from build123d import *

# Parameters (mm, degrees)
SKETCH_R           = 0.75
SKETCH_R_2         = 0.6
PAD_DEPTH          = 4.8
PAD_DEPTH_BACK     = 0.8
SKETCH001_R        = 3.5
SKETCH001_R_2      = 0.6
PAD001_DEPTH       = 0.8
POCKET_DEPTH       = 24.348308
POLARPATTERN_COUNT = 4
SKETCH003_R        = 1.5
SKETCH003_R_2      = 0.6
PAD002_DEPTH       = 0.2


with BuildPart() as part:
    # Sketch → Pad (new body, two sides)
    with BuildSketch(Plane.XY) as pad_sk:
        Circle(SKETCH_R)
        Circle(SKETCH_R_2, mode=Mode.SUBTRACT)
    extrude(amount=PAD_DEPTH)
    extrude(pad_sk.sketch, amount=-PAD_DEPTH_BACK)

    # Sketch001 → Pad001 (join)
    with BuildSketch(Plane.XY):
        Circle(SKETCH001_R)
        Circle(SKETCH001_R_2, mode=Mode.SUBTRACT)
    extrude(amount=PAD001_DEPTH)

    # Sketch002 (on Face8 of Pad001) → Pocket (cut, through all)
    with BuildSketch(Plane.XY.offset(0.8)):
        with BuildLine():
            Line((-0.5, 3.75), (0.5, 3.75))
            Line((0.5, 3.75), (0.5, 2.25))
            ThreePointArc((-0.5, 2.25), (0, 1.75), (0.5, 2.25))
            Line((-0.5, 2.25), (-0.5, 3.75))
        make_face()
    pocket = extrude(amount=-POCKET_DEPTH, mode=Mode.SUBTRACT)

    # PolarPattern: Pocket ×4 about axis
    polarpattern_axis = Axis((0, 0, 0.8), (0, 0, 1))
    for i in range(1, POLARPATTERN_COUNT):
        add(pocket.rotate(polarpattern_axis, i * 360 / POLARPATTERN_COUNT), mode=Mode.SUBTRACT)

    # Sketch003 (on Face23 of PolarPattern) → Pad002 (join)
    with BuildSketch(Plane.XY.offset(0.8)):
        Circle(SKETCH003_R)
        Circle(SKETCH003_R_2, mode=Mode.SUBTRACT)
    extrude(amount=PAD002_DEPTH)


solid = part.part
Geometry check sheet. Reference: the model listing, model coordinates, mm. A direction names the side the tool comes from. Round coordinates to 2 decimals unless told otherwise and drop trailing zeros. Loops run counter-clockwise (first coordinate to the right, second up) from the corner with the lowest first, then second, coordinate; pieces in that order, holes last. Notation, with made-up numbers: (58.5, 68) - (109.5, 68) arc R23 ccw to (109.5, 79) - close; hole circle Ø7 at (58.25, -2). An arc over 180 degrees is marked (long way). One line per question, with ' | ' between items. Start each with the question number.
1. Depth check by flat-ended pin: pin 1 (1 mm diameter, centred on x = 1, z = 3, fed in from -Y); pin 2 (0.6 mm diameter, centred on x = 3, z = 0.5, fed in from +Y); pin 3 (0.9 mm diameter, centred on y = -3, z = 0.5, fed in from -X); pin 4 (3.5 mm diameter, centred on x = 0.5, y = 1.5, fed in from -Z). Enter the tip coordinate at first touch or a pass-through.
2. Draft check along Y on faces 1 (the face through (1.5, -0.7, 0.8)), 2 (the face through (-0.6, 0, 2)), 3 (the face through (-0.75, 0.03, -0.39)), 4 (the face through (-2.5, -2.45, 0.39)). Enter one of: released by +Y, released by -Y, zero draft, split by the parting line, or undercut.
3. Cross-section at D-D on x = -2.5. Record the cut outline in (y, z), then the cut area to 3 significant figures.
4. Tool access check on faces 5 (the face through (-1, 0, 1)), 6 (the face through (-2.45, 2.5, 0.39)). Record the directions out of +Z, -Z, +X, -X, +Y, -Y that give a thin tool (end or side, any length) a straight path to the whole face; none if there is none.
5. Cross-section at A-A on x = 0. Record the cut outline in (y, z).
6. Scan lines: line 1 (Z direction, x = 1.75, y = 0.25); line 2 (Z direction, x = 0, y = -1.25); line 3 (Y direction, x = 0.5, z = 1.95). Record each from-to range of solid material in increasing order. Write a range as [from, to].
7. Cross-section at C-C on z = 4.35. Record the cut outline in (x, y).
Taken from the geometry:
1) pin 1: y = -0.56 | pin 2: y = 2.23 | pin 3: x = -2.4 | pin 4: z = -0.8
2) face 1: zero draft | face 2: undercut | face 3: split by the parting line | face 4: released by -Y
3) outline: (-2.45, 0) - (-0.5, 0) - (-0.5, 0.8) - (-2.45, 0.8) - close; (0.5, 0) - (2.45, 0) - (2.45, 0.8) - (0.5, 0.8) - close | area: 3.12 mm²
4) face 5: +Z | face 6: +Z, -Z, -X, +Y
5) outline: (-1.75, 0) - (-0.75, 0) - (-0.75, -0.8) - (-0.6, -0.8) - (-0.6, 4.8) - (-0.75, 4.8) - (-0.75, 1) - (-1.5, 1) - (-1.5, 0.8) - (-1.75, 0.8) - close; (0.6, -0.8) - (0.75, -0.8) - (0.75, 0) - (1.75, 0) - (1.75, 0.8) - (1.5, 0.8) - (1.5, 1) - (0.75, 1) - (0.75, 4.8) - (0.6, 4.8) - close
6) line 1: [0, 0.8] | line 2: [0, 1] | line 3: [-0.56, -0.33], [0.33, 0.56]
7) outline: circle Ø1.5 at (0, 0); hole circle Ø1.2 at (0, 0)
